Read the model definition and answer for the solid it produces. Units are mm, in the model's axes. A direction names the side the tool comes from. Give positions to 0.01 mm unless a question says otherwise; leave off trailing zeros. Order: outer loops, then holes, each group sorted by start corner. A loop starts at its lowest first (then second) coordinate and runs counter-clockwise, first axis right, second up. Notation, with made-up numbers: M 46.5,45.5 L 70.5,45.5 A26 ccw 70.5,82.5 Z; hole C -3.75,-11.75 d5. An arc over 180 degrees is marked long. Write item = value, one per line. Start each with the question number.
from build123d import *

# Parameters (mm, degrees)
F0_W     = 34.514117986
F0_H     = 55.7645447552
F1_DEPTH = 25.4
F2_R     = 3.8523335732
F3_DEPTH = 55.7655447552
F4_W     = 28.238822706
F4_H     = 49.3466292974
F5_DEPTH = 25.401
F6_W     = 13.4063102305
F6_H     = 13.5625138223
F7_DEPTH = 34.515117986


with BuildPart() as f1:
    # F0 (on Top) → F1 (new body)
    with BuildSketch(Plane.XY):
        with Locations((17.257058993, 27.8822723776)):
            Rectangle(F0_W, F0_H)
    extrude(amount=F1_DEPTH)

    # F2 (on face) → F3 (cut, through all)
    with BuildSketch(Plane.XZ):
        with Locations((16.971334815, 12.0531069115)):
            Circle(F2_R)
    extrude(amount=-F3_DEPTH, mode=Mode.SUBTRACT)

    # F4 (on face) → F5 (cut, through all)
    with BuildSketch(Plane.XY.offset(25.4)):
        with Locations((17.2570585273, 27.9535820009)):
            Rectangle(F4_W, F4_H)
    extrude(amount=-F5_DEPTH, mode=Mode.SUBTRACT)

    # F6 (on face) → F7 (cut, through all)
    with BuildSketch(Plane(origin=(0, 0, 0), x_dir=(0, -1, 0), z_dir=(-1, 0, 0))):
        with Locations((-27.8109628707, 18.6187430888)):
            Rectangle(F6_W, F6_H)
    extrude(amount=-F7_DEPTH, mode=Mode.SUBTRACT)


solid = f1.part
1) Find section D-D on x = 14. Determine the outline of the cut face in (y, z).
2) Find the intervals of material crossed by probe 1 along X at (y, z) = (5, 16.25); probe 2 along Y at (x, z) = (7, 22.5); probe 3 along Y at (x, z) = (31.5, 18.25), in increasing order. Write a range as [from, to].
3) This flat-tipped pin is pushed along its axis until it touches: P1, Ø1.6, axis at x = 1, y = 28.5, coming from the +Z side. Where does it stop, or does it pass through?
4) Find section A-A on y = 40. Determine the outline of the cut face in (x, z).
5) For faces 5 (the face through (33, 21.108, 19)), 6 (the face through (14, 3.28, 16)), 7 (the face through (34.514, 27, 10)), determine the directions among +Z, -Z, +X, -X, +Y, -Y from which every point of the face is accessible in a straight line to the end or side of a thin tool.
6) For a pull along Y with two mould halves and no side action, classify faces 1 (the face through (2, 28, 11.837)), 2 (the face through (21, 55.765, 13)), 3 (the face through (2, 21.108, 19)), 4 (the face through (16.47, 54.174, 15.873)) as pulls with the +Y half, pulls with the -Y half, needs draft (parallel to the pull), parting line crosses it, or undercut.
7) Find section B-B on z = 16.5. Determine the outline of the cut face in (x, y).
8) Find section C-C on x = 30.5. Determine the outline of the cut face in (y, z).
Numbers:
q1.outline = M 0,0 L 3.28,0 L 3.28,9.6 L 0,9.6 Z; M 0,14.5 L 3.28,14.5 L 3.28,25.4 L 0,25.4 Z; M 52.63,0 L 55.76,0 L 55.76,9.6 L 52.63,9.6 Z; M 52.63,14.5 L 55.76,14.5 L 55.76,25.4 L 52.63,25.4 Z
q2.probe_1 = [0, 3.14], [31.38, 34.51]
q2.probe_2 = [0, 3.28], [52.63, 55.76]
q2.probe_3 = [0, 21.11], [34.51, 55.76]
q3.P1 = 11.84
q4.outline = M 0,0 L 3.14,0 L 3.14,25.4 L 0,25.4 Z; M 31.38,0 L 34.51,0 L 34.51,25.4 L 31.38,25.4 Z
q5.face_5 = +Z, +X, -X
q5.face_6 = +Z, -Z
q5.face_7 = +Z, -Z, +X, +Y, -Y
q6.face_1 = undercut
q6.face_2 = pulls with the +Y half
q6.face_3 = undercut
q6.face_4 = needs draft
q7.outline = M 0,0 L 34.51,0 L 34.51,21.11 L 31.38,21.11 L 31.38,3.28 L 3.14,3.28 L 3.14,21.11 L 0,21.11 Z; M 0,34.51 L 3.14,34.51 L 3.14,52.63 L 31.38,52.63 L 31.38,34.51 L 34.51,34.51 L 34.51,55.76 L 0,55.76 Z
q8.outline = M 0,0 L 3.28,0 L 3.28,25.4 L 0,25.4 Z; M 52.63,0 L 55.76,0 L 55.76,25.4 L 52.63,25.4 Z
